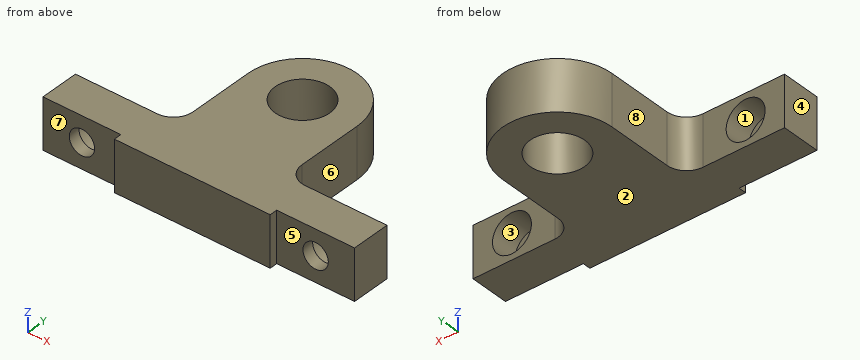
Autodesk Inventor part; units mm, degrees
ref_plane "YZ Plane" through (0, 0, 0) normal (1, 0, 0) x (0, 1, 0)
ref_plane "XZ Plane" through (0, 0, 0) normal (0, 1, 0) x (-1, 0, 0)
ref_plane "XY Plane" through (0, 0, 0) normal (0, 0, 1) x (1, 0, 0)
sketch "Sketch1" plane through (0, 0, 0) normal (0, 0, 1) x (1, 0, 0)
  line L0 (0, 0) -> (80, 0)
  line L1 (80, 0) -> (80, 48)
  line L2 (80, 48) -> (0, 48)
  line L3 (0, 48) -> (0, 0)
  dimension "d0" = 80
  dimension "d1" = 48
extrude "Extrusion1" add sketch "Sketch1" along normal blind 13
sketch "Sketch2" plane through (0, 0, 13) normal (0, 0, 1) x (1, 0, 0)
  line L0 (80, 0) -> (0, 0)
  line L1 (80, 48) -> (80, 0)
  point P0 (40, 34)
  dimension "d4" = 34
  dimension "d5" = 40
hole "Hole1" at (40, 34, 13) direction (0, 0, -1) diameter 14 depth 13 tip angle 118
sketch "Sketch3" plane through (0, 0, 13) normal (0, 0, 1) x (1, 0, 0)
  circle A0 centre (40, 34) radius 7
  line L0 (0, 0) -> (0, 48)
  line L1 (80, 0) -> (0, 0)
  line L2 (80, 48) -> (80, 0)
  line L3 (0, 48) -> (80, 48)
  arc A1 (54, 34) -> (26, 34) centre (40, 34) ccw
  line L4 (54, 34) -> (54, 12)
  line L5 (26, 34) -> (26, 12)
  line L6 (0, 12) -> (26, 12)
  line L7 (54, 12) -> (80, 12)
  dimension "d14" = 12
  dimension "d15" = 12
  dimension "d16" = 26
extrude "Extrusion2" cut sketch "Sketch3" against normal blind 13 contours L0 L3 A1 L5 L6 | L7 L4 A1 L3 L2
sketch "Sketch4" plane through (0, 0, 13) normal (0, 0, 1) x (1, 0, 0)
  line L0 (0, 0) -> (0, 12)
  line L1 (80, 0) -> (0, 0)
  line L2 (80, 12) -> (80, 0)
  line L3 (0, 2) -> (20, 2)
  line L4 (20, 2) -> (20, 0)
  line L5 (20, 0) -> (0, 0)
  line L6 (0, 0) -> (0, 2)
  line L7 (60, 0) -> (80, 0)
  line L8 (80, 0) -> (80, 2)
  line L9 (80, 2) -> (60, 2)
  line L10 (60, 2) -> (60, 0)
  dimension "d19" = 2
  dimension "d20" = 2
  dimension "d21" = 20
  dimension "d22" = 20
extrude "Extrusion3" cut sketch "Sketch4" against normal blind 13
sketch "Sketch5" plane through (0, 12, 13) normal (0, 1, 0) x (1, 0, 0)
  line L0 (0, 0) -> (0, 13)
  line L1 (26, 0) -> (0, 0)
  line L2 (54, 13) -> (80, 13)
  line L3 (54, 0) -> (54, 13)
  line L4 (80, 0) -> (54, 0)
  line L5 (80, 13) -> (80, 0)
  point P0 (10, 6.5)
  point P1 (70, 6.5)
  dimension "d25" = 60
  dimension "d26" = 10
  dimension "d27" = 6.5
hole "Hole2" at (10, 12, 6.5) at (70, 12, 6.5) direction (0, -1, 0) diameter 6.5 depth 10 tip angle 118 counterbore diameter 10 counterbore depth 7
fillet "Fillet1" radius 5 2 edges at (54, 12, 6.5) (26, 12, 6.5)
properties part number "MANCAL DA BETONEIRA(26)" material "Carbon Steel"
For this review, take the finished solid that the model builds, in its own axes (mm). Face numbers are marked on the shaded views. A direction names the side the tool comes from. Give positions to 0.01 mm unless a question says otherwise; leave off trailing zeros. Write each loop counter-clockwise with the first axis right and the second up, starting at its lowest first coordinate (ties: lowest second). Pieces come first, ordered by that corner, then holes. Notation, with made-up numbers: M 18,88 L 71,88 A20 ccw 71,116 Z; hole C 47.5,-30.75 d6. An arc over 180 degrees is marked long. Answer as a JSON object with one key per item and string values. Group by question number.
Item 1: Tool access review of the marked faces 5, 6, 7 and 8: name each direction out of +Z, -Z, +X, -X, +Y, -Y from which nothing blocks a thin tool from reaching the whole face with its end or side.
Item 2: For pin 1 Ø1.6 at (y, z) = (0.5, 6.5) entering from -X; pin 2 Ø1 at (y, z) = (24, 7) entering from +X; pin 3 Ø2 at (y, z) = (14.5, 6.5) entering from +X; pin 4 Ø4 at (x, y) = (46, 14) entering from -Z, all flat-tipped, find the tip position at first contact; note any pin that passes through.
Item 3: Consider section D-D on x = 40. Write out the cut boundary in (y, z), plus the area to 3 significant figures.
Item 4: Draft analysis for pull direction Z (two halves, no side actions). For the marked faces 1, 2, 3 and 4, state which applies: +Z half, -Z half, draft (parallel to the pull), parting line (faces both ways), or undercut.
Item 5: Consider section C-C on y = 40. Write out the cut boundary in (x, z), plus the area to 3 significant figures.
Item 6: Consider section B-B on x = 10. Write out the cut boundary in (y, z).
Item 7: Consider section A-A on z = 6.5. Count the separate pieces of the cut face and the enclosed holes in it, plus the area to 3 significant figures.
Item 8: For probe 1 along X at (y, z) = (9.25, 6.5); probe 2 along X at (y, z) = (34, 5.5); probe 3 along X at (y, z) = (3.3, 6.5), list the stretches that pass through material, from the lowest coordinate up. Write a range as [from, to].
Check result:
{
 "1": {"face 5": "+Z, -Z, +X, -Y", "face 6": "+Z, -Z, +X, +Y", "face 7": "+Z, -Z, -X, -Y", "face 8": "+Z, -Z, -X, +Y"},
 "2": {"pin 1": "stops at x = 20", "pin 2": "stops at x = 54", "pin 3": "stops at x = 55.43", "pin 4": "stops at z = 0"},
 "3": {"outline": "M 0,0 L 27,0 L 27,13 L 0,13 Z; M 41,0 L 48,0 L 48,13 L 41,13 Z", "area": "442 mm^2"},
 "4": {"face 1": "undercut", "face 2": "-Z half", "face 3": "undercut", "face 4": "draft"},
 "5": {"outline": "M 27.35,0 L 36.39,0 L 36.39,13 L 27.35,13 Z; M 43.61,0 L 52.65,0 L 52.65,13 L 43.61,13 Z", "area": "235 mm^2"},
 "6": {"outline": "M 2,0 L 12,0 L 12,1.5 L 5,1.5 L 5,3.25 L 2,3.25 Z; M 2,9.75 L 5,9.75 L 5,11.5 L 12,11.5 L 12,13 L 2,13 Z"},
 "7": {"separate pieces": "3", "enclosed holes": "1", "area": "1,480 mm^2"},
 "8": {"probe 1": "x = [0, 5], [15, 65], [75, 80]", "probe 2": "x = [26, 33], [47, 54]", "probe 3": "x = [0, 6.75], [13.25, 66.75], [73.25, 80]"}
}
